```python
from build123d import *

# Parameters (mm, degrees)
SKETCH_1_W               = 58
SKETCH_1_H               = 58
EXTRUDE_1_DEPTH          = 2.5
SKETCH_2_W               = 57
SKETCH_2_H               = 57
CUT_EXTRUDE_7_DEPTH      = 1
CUT_EXTRUDE_7_DEPTH_BACK = 3.5
SKETCH_5_W               = 1.4427437
SKETCH_5_H               = 2.5
CUT_EXTRUDE_8_DEPTH      = 1.5
SKETCH_6_W               = 1.3
SKETCH_6_H               = 1.3
EXTRUDE_5_DEPTH          = 0.8
FILLET_4_R               = 2
FILLET_5_R               = 2
SKETCH_8_W               = 1.3
SKETCH_8_H               = 1.3
EXTRUDE_6_DEPTH          = 0.8
SKETCH_10_W              = 1.3
SKETCH_10_H              = 1.3
EXTRUDE_8_DEPTH          = 0.8
SKETCH_12_W              = 1.3
SKETCH_12_H              = 1.3
EXTRUDE_9_DEPTH          = 0.8


with BuildPart() as part:
    # 草图1 → 凸台-拉伸1 (new body)
    with BuildSketch(Plane(origin=(0, 0, 0), x_dir=(1, 0, 0), z_dir=(0, 1, 0))):
        Rectangle(SKETCH_1_W, SKETCH_1_H)
    extrude(amount=EXTRUDE_1_DEPTH)

    # 草图2 → 切除-拉伸7 (cut, two sides)
    with BuildSketch(Plane(origin=(0, 2.5, 0), x_dir=(1, 0, 0), z_dir=(0, 1, 0))) as cut_extrude_7_sk:
        Rectangle(SKETCH_2_W, SKETCH_2_H)
    extrude(amount=CUT_EXTRUDE_7_DEPTH, mode=Mode.SUBTRACT)
    extrude(cut_extrude_7_sk.sketch, amount=-CUT_EXTRUDE_7_DEPTH_BACK, mode=Mode.SUBTRACT)

    # 草图5 → 切除-拉伸8 (cut, through all)
    with BuildSketch(Plane.XY.offset(-28.5)):
        with Locations((27.77862815, 1.25)):
            Rectangle(SKETCH_5_W, SKETCH_5_H)
    extrude(amount=-CUT_EXTRUDE_8_DEPTH, mode=Mode.SUBTRACT)

    # 草图6 → 凸台-拉伸5 (add)
    with BuildSketch(Plane.XY.offset(-28.5)):
        with Locations((14.7572563, 1.25)):
            Rectangle(SKETCH_6_W, SKETCH_6_H)
        with Locations((23.0572563, 1.25)):
            Rectangle(SKETCH_6_W, SKETCH_6_H)
        with Locations((6.4572563, 1.25)):
            Rectangle(SKETCH_6_W, SKETCH_6_H)
        with Locations((-1.8427437, 1.25)):
            Rectangle(SKETCH_6_W, SKETCH_6_H)
        with Locations((-10.1427437, 1.25)):
            Rectangle(SKETCH_6_W, SKETCH_6_H)
        with Locations((-18.4427437, 1.25)):
            Rectangle(SKETCH_6_W, SKETCH_6_H)
    extrude(amount=EXTRUDE_5_DEPTH)

    # 圆角4
    fillet_4_edges = [part.edges().sort_by_distance(p)[0] for p in [
        (28.5, 1.25, 28.5),
        (-28.5, 1.25, 28.5),
        (-28.5, 1.25, -28.5),
    ]]
    fillet(fillet_4_edges, radius=FILLET_4_R)

    # 圆角5
    fillet_5_edges = [part.edges().sort_by_distance(p)[0] for p in [
        (29, 1.25, 29),
        (-29, 1.25, 29),
        (-29, 1.25, -29),
    ]]
    fillet(fillet_5_edges, radius=FILLET_5_R)

    # 草图8 → 凸台-拉伸6 (add)
    with BuildSketch(Plane(origin=(-28.5, 0, 0), x_dir=(0, 0, -1), z_dir=(1, 0, 0))):
        with Locations((17.2572563, 1.25)):
            Rectangle(SKETCH_8_W, SKETCH_8_H)
        with Locations((25.5572563, 1.25)):
            Rectangle(SKETCH_8_W, SKETCH_8_H)
        with Locations((8.9572563, 1.25)):
            Rectangle(SKETCH_8_W, SKETCH_8_H)
        with Locations((0.6572563, 1.25)):
            Rectangle(SKETCH_8_W, SKETCH_8_H)
        with Locations((-7.6427437, 1.25)):
            Rectangle(SKETCH_8_W, SKETCH_8_H)
        with Locations((-15.9427437, 1.25)):
            Rectangle(SKETCH_8_W, SKETCH_8_H)
        with Locations((-24.2427437, 1.25)):
            Rectangle(SKETCH_8_W, SKETCH_8_H)
    extrude(amount=EXTRUDE_6_DEPTH)

    # 草图10 → 凸台-拉伸8 (add)
    with BuildSketch(Plane(origin=(0, 0, 28.5), x_dir=(-1, 0, 0), z_dir=(0, 0, -1))):
        with Locations((19.7572563, 1.25)):
            Rectangle(SKETCH_10_W, SKETCH_10_H)
        with Locations((11.4572563, 1.25)):
            Rectangle(SKETCH_10_W, SKETCH_10_H)
        with Locations((3.1572563, 1.25)):
            Rectangle(SKETCH_10_W, SKETCH_10_H)
        with Locations((-5.1427437, 1.25)):
            Rectangle(SKETCH_10_W, SKETCH_10_H)
        with Locations((-13.4427437, 1.25)):
            Rectangle(SKETCH_10_W, SKETCH_10_H)
        with Locations((-21.7427437, 1.25)):
            Rectangle(SKETCH_10_W, SKETCH_10_H)
    extrude(amount=EXTRUDE_8_DEPTH)

    # 草图12 → 凸台-拉伸9 (add)
    with BuildSketch(Plane.ZY.offset(-28.5)):
        with Locations((20.1072563, 1.25)):
            Rectangle(SKETCH_12_W, SKETCH_12_H)
        with Locations((11.8072563, 1.25)):
            Rectangle(SKETCH_12_W, SKETCH_12_H)
        with Locations((3.5072563, 1.25)):
            Rectangle(SKETCH_12_W, SKETCH_12_H)
        with Locations((-4.7927437, 1.25)):
            Rectangle(SKETCH_12_W, SKETCH_12_H)
        with Locations((-13.0927437, 1.25)):
            Rectangle(SKETCH_12_W, SKETCH_12_H)
        with Locations((-21.3927437, 1.25)):
            Rectangle(SKETCH_12_W, SKETCH_12_H)
    extrude(amount=EXTRUDE_9_DEPTH)


solid = part.part
```
Design review of the part built by this model. Coordinates are the model's own, in mm. A direction names the side the tool comes from. Give positions to 0.01 mm unless a question says otherwise; leave off trailing zeros. Loops run counter-clockwise (first coordinate to the right, second up) from the corner with the lowest first, then second, coordinate; pieces in that order, holes last. Notation, with made-up numbers: M -9.5,32 L 30.5,32 A34 cw 30.5,63 Z; hole C 37,31 d9. An arc over 180 degrees is marked long. Return JSON: item names as keys, results as strings. Group by question number.
Item 1: Mouldability with a two-part tool opening along Z and no side actions: class faces 3 (the flat face through (27.7, 1.3, 3.5)), 4 (the flat face through (-27.7, 1, 24)) as released by +Z, released by -Z, zero draft, split by the parting line, or undercut.
Item 2: For probe 1 along Z at (x, y) = (17.5, 1.25); probe 2 along X at (y, z) = (1.1, 19.5), list the stretches that pass through material, from the lowest coordinate up.
Item 3: We need section A-A (x = -5.5). Give the boundary of the cut face in (y, z), and give its area (3 significant figures).
Item 4: Insertion check: pin 1 Ø0.6 at (x, z) = (28, -4.5) entering from +Y; pin 2 Ø0.9 at (y, z) = (1.5, 28) entering from +X. Each pin has a flat end and moves straight along its axis. Give the tip position at first contact, or say it passes through.
Item 5: Tool access review of faces 1 (the flat face through (27.7, 1, -5)), 2 (the flat face through (-3, 1, 27.7)): name each direction out of +Z, -Z, +X, -X, +Y, -Y from which nothing blocks a thin tool from reaching the whole face with its end or side.
Output:
{
 "1": {"face 3": "zero draft", "face 4": "undercut"},
 "2": {"probe 1": "z = -29 to -28.5, 28.5 to 29", "probe 2": "x = -29 to -28.5, 27.7 to 29"},
 "3": {"outline": "M 0,-29 L 2.5,-29 L 2.5,-28.5 L 0,-28.5 Z; M 0,28.5 L 2.5,28.5 L 2.5,29 L 0,29 Z", "area": "2.50 mm^2"},
 "4": {"pin 1": "stops at y = 1.9", "pin 2": "stops at x = 28.92"},
 "5": {"face 1": "-Z, +Y, -Y", "face 2": "+Y, -Y"}
}
